For this review, take the finished solid that the model builds, in its own axes (mm). A direction names the side the tool comes from. Give positions to 0.01 mm unless a question says otherwise; leave off trailing zeros. Loops run counter-clockwise (first coordinate to the right, second up) from the corner with the lowest first, then second, coordinate; pieces in that order, holes last. Notation, with made-up numbers: (60, 26) -> (100, 26) arc R20 ccw to (100, 39) -> close; hole circle Ø6 at (5, 44). An arc over 180 degrees is marked (long way). One line per question, with ' | ' between items. Start each with the question number.
(1) Consider section A-A (z = 0). Write out the cut boundary in (x, y).
(2) Tool access review of faces 5 (the flat face through (3, 28, 0)), 6 (the flat face through (3.4, 27, 0.1)): name each direction out of +Z, -Z, +X, -X, +Y, -Y from which nothing blocks a thin tool from reaching the whole face with its end or side.
(3) Consider section C-C (x = -2.5). Write out the cut boundary in (y, z), and give its area (3 significant figures).
(4) Wall thickness on probe 1 along Z at (x, y) = (0, 14); probe 2 along Z at (x, y) = (-4.75, 5); probe 3 along X at (y, z) = (24, 5.75): over which ranges is each line inside the solid? List them lowest first.
(5) Consider section D-D (z = 3.75). Write out the cut boundary in (x, y).
(6) Draft analysis for pull direction X (two halves, no side actions). For faces 1 (the flat face through (-4.44, 28.52, 0.13)), 2 (the cylindrical face through (8.584, 14.79, 2.703)), 3 (the cylindrical face through (-1.73, 13.31, -7.81)), 4 (the flat face through (4.44, 28.52, 0.13)), state which applies: +X half, -X half, draft (parallel to the pull), parting line (faces both ways), or undercut.
(7) Consider section B-B (y = 14). Write out the cut boundary in (x, z).
(8) Insertion check: P1, Ø1, axis at y = 19, z = 5.5, coming from the +X side; P2, Ø8, axis at x = 4.5, y = 11.5, coming from the -Z side; P3, Ø3, axis at x = 6.5, z = 5, coming from the +Y side; P4, Ø4, axis at y = 23.5, z = -1, coming from the -X side. Each pin has a flat end and moves straight along its axis. Give the tip position at first contact, or say it passes through.
from build123d import *

# Parameters (mm, degrees)
BOSS_EXTRUDE3_DEPTH      = 9
BOSS_EXTRUDE3_DEPTH_BACK = 9
SKETCH7_R                = 14.642288151
SKETCH7_R_2              = 9
CUT_EXTRUDE3_DEPTH       = 32
SKETCH8_W                = 6
SKETCH8_H                = 6
CUT_EXTRUDE4_DEPTH       = 32
SKETCH9_R                = 8
CUT_EXTRUDE5_DEPTH       = 27


with BuildPart() as part:
    # Sketch1 → Revolve4 (revolve)
    with BuildSketch(Plane.XY):
        Polygon((0, 27), (9, 27), (9, 24.588457268), (9, 0), (0, 0), align=None)
    revolve(axis=Axis((0, 0, 0), (0, 1, 0)))

    # Sketch6 → Boss-Extrude3 (add, two sides)
    with BuildSketch(Plane.XY) as boss_extrude3_sk:
        Polygon((0, 27), (0, 30), (9, 27), align=None)
        Polygon((0, 30), (-9, 27), (0, 27), align=None)
    extrude(amount=BOSS_EXTRUDE3_DEPTH)
    extrude(boss_extrude3_sk.sketch, amount=-BOSS_EXTRUDE3_DEPTH_BACK)

    # Sketch7 → Cut-Extrude3 (cut)
    with BuildSketch(Plane.XZ):
        Circle(SKETCH7_R)
        Circle(SKETCH7_R_2, mode=Mode.SUBTRACT)
    extrude(amount=-CUT_EXTRUDE3_DEPTH, mode=Mode.SUBTRACT)

    # Sketch8 → Cut-Extrude4 (cut)
    with BuildSketch(Plane(origin=(0, 0, 0), x_dir=(-1, 0, 0), z_dir=(0, -1, 0))):
        Rectangle(SKETCH8_W, SKETCH8_H)
    extrude(amount=-CUT_EXTRUDE4_DEPTH, mode=Mode.SUBTRACT)

    # Sketch9 → Cut-Extrude5 (cut)
    with BuildSketch(Plane.XZ):
        Circle(SKETCH9_R)
    extrude(amount=-CUT_EXTRUDE5_DEPTH, mode=Mode.SUBTRACT)


solid = part.part
A:
1) outline: (-9, 0) -> (-8, 0) -> (-8, 27) -> (-3, 27) -> (-3, 29) -> (-9, 27) -> close; (3, 27) -> (8, 27) -> (8, 0) -> (9, 0) -> (9, 27) -> (3, 29) -> close
2) face 5: +Y, -Y | face 6: -Y
3) outline: (0, -8.65) -> (29.17, -8.65) -> (29.17, -3) -> (27, -3) -> (27, -7.6) -> (0, -7.6) -> close; (0, 7.6) -> (27, 7.6) -> (27, 3) -> (29.17, 3) -> (29.17, 8.65) -> (0, 8.65) -> close | area: 81.0 mm^2
4) probe 1: z = -9 to -8, 8 to 9 | probe 2: z = -7.64 to -6.44, 6.44 to 7.64 | probe 3: x = -6.92 to -5.56, 5.56 to 6.92
5) outline: (-8.18, 0) -> (-7.07, 0) -> (-7.07, 27) -> (7.07, 27) -> (7.07, 0) -> (8.18, 0) -> (8.18, 27.27) -> (0, 30) -> (-8.18, 27.27) -> close
6) face 1: -X half | face 2: parting line | face 3: undercut | face 4: +X half
7) outline: circle Ø18 at (0, 0); hole circle Ø16 at (0, 0)
8) P1: stops at x = 7.48 | P2: stops at z = -8.99 | P3: stops at y = 28.33 | P4: stops at x = -9
